Input: part model. Units: mm. Frame: model coordinates. A direction names the side the tool comes from. Give positions to 0.01 mm unless a question says otherwise; leave off trailing zeros. Loops run counter-clockwise (first coordinate to the right, second up) from the corner with the lowest first, then second, coordinate; pieces in that order, holes last. Notation, with made-up numbers: (85, 5) - (122, 5) arc R17 cw to (122, 19) - close; hole circle Ø4 at (59.5, 81.25). An arc over 180 degrees is marked (long way). One line per item, written item: value.
from build123d import *

# Parameters (mm, degrees)
F0_R     = 3.048
F0_R_2   = 2.54
F1_DEPTH = 3.937
F2_R     = 3.0417071759
F3_DEPTH = 0.635
F4_R     = 3.048
F5_DEPTH = 0.635
F6_SIZE2 = 0.50799
F6_SIZE  = 0.50799
F7_SIZE2 = 0.50799
F7_SIZE  = 0.50799


# Not quite as in the source:
# - a fillet or chamfer is up to 0.001 mm smaller than in the source, because OpenCascade refuses the exact size


with BuildPart() as f1:
    # F0 (on Top) → F1 (new body, symmetric)
    with BuildSketch(Plane.XY):
        with BuildLine():
            ThreePointArc((-40.9946195992, 14.3710068385), (-42.0464330806, 16.9103092103), (-44.5857354524, 17.9621226917))
            ThreePointArc((-44.5857354524, 17.9621226917), (-48.1768513056, 14.3710068385), (-44.5857354524, 10.7798909853))
            ThreePointArc((-44.5857354524, 10.7798909853), (-42.0464330806, 11.8317044667), (-40.9946195992, 14.3710068385))
        make_face()
        with Locations((-44.5857354524, 14.3710068385)):
            Circle(F0_R, mode=Mode.SUBTRACT)
        with BuildLine():
            ThreePointArc((-49.1226195992, 14.3710068385), (-50.1744330806, 16.9103092103), (-52.7137354524, 17.9621226917))
            ThreePointArc((-52.7137354524, 17.9621226917), (-56.3048513056, 14.3710068385), (-52.7137354524, 10.7798909853))
            ThreePointArc((-52.7137354524, 10.7798909853), (-50.1744330806, 11.8317044667), (-49.1226195992, 14.3710068385))
        make_face()
        with Locations((-52.7137354524, 14.3710068385)):
            Circle(F0_R, mode=Mode.SUBTRACT)
        with BuildLine():
            ThreePointArc((-32.8666195992, 14.3710068385), (-33.9184330806, 16.9103092103), (-36.4577354524, 17.9621226917))
            ThreePointArc((-36.4577354524, 17.9621226917), (-40.0488513056, 14.3710068385), (-36.4577354524, 10.7798909853))
            ThreePointArc((-36.4577354524, 10.7798909853), (-33.9184330806, 11.8317044667), (-32.8666195992, 14.3710068385))
        make_face()
        with Locations((-36.4577354524, 14.3710068385)):
            Circle(F0_R, mode=Mode.SUBTRACT)
        with BuildLine():
            ThreePointArc((-24.7386195992, 14.3710068385), (-25.7904330806, 16.9103092103), (-28.3297354524, 17.9621226917))
            ThreePointArc((-28.3297354524, 17.9621226917), (-31.9208513056, 14.3710068385), (-28.3297354524, 10.7798909853))
            ThreePointArc((-28.3297354524, 10.7798909853), (-25.7904330806, 11.8317044667), (-24.7386195992, 14.3710068385))
        make_face()
        with Locations((-28.3297354524, 14.3710068385)):
            Circle(F0_R, mode=Mode.SUBTRACT)
        with BuildLine():
            ThreePointArc((-60.8417354524, 10.7798909853), (-58.3024330806, 11.8317044667), (-57.2506195992, 14.3710068385))
            ThreePointArc((-57.2506195992, 14.3710068385), (-58.3024330806, 16.9103092103), (-60.8417354524, 17.9621226917))
            ThreePointArc((-60.8417354524, 17.9621226917), (-64.4328513056, 14.3710068385), (-60.8417354524, 10.7798909853))
        make_face()
        with Locations((-60.8417354524, 14.3710068385)):
            Circle(F0_R, mode=Mode.SUBTRACT)
        with Locations((-44.5857354524, 14.3710068385)):
            Circle(F0_R)
        with Locations((-44.5857354524, 14.3710068385)):
            Circle(F0_R_2, mode=Mode.SUBTRACT)
        with Locations((-36.4577354524, 14.3710068385)):
            Circle(F0_R)
        with Locations((-36.4577354524, 14.3710068385)):
            Circle(F0_R_2, mode=Mode.SUBTRACT)
        with Locations((-52.7137354524, 14.3710068385)):
            Circle(F0_R)
        with Locations((-52.7137354524, 14.3710068385)):
            Circle(F0_R_2, mode=Mode.SUBTRACT)
        with Locations((-28.3297354524, 14.3710068385)):
            Circle(F0_R)
        with Locations((-28.3297354524, 14.3710068385)):
            Circle(F0_R_2, mode=Mode.SUBTRACT)
        with Locations((-60.8417354524, 14.3710068385)):
            Circle(F0_R)
        with Locations((-60.8417354524, 14.3710068385)):
            Circle(F0_R_2, mode=Mode.SUBTRACT)
        with BuildLine():
            ThreePointArc((-60.8417354524, 17.9621226917), (-58.3024330806, 16.9103092103), (-57.2506195992, 14.3710068385))
            ThreePointArc((-57.2506195992, 14.3710068385), (-58.3024330806, 11.8317044667), (-60.8417354524, 10.7798909853))
            Line((-60.8417354524, 10.7798909853), (-52.7137354524, 10.7798909853))
            ThreePointArc((-52.7137354524, 10.7798909853), (-56.3048513056, 14.3710068385), (-52.7137354524, 17.9621226917))
            Line((-52.7137354524, 17.9621226917), (-60.8417354524, 17.9621226917))
        make_face()
        with BuildLine():
            Line((-44.5857354524, 17.9621226917), (-52.7137354524, 17.9621226917))
            ThreePointArc((-52.7137354524, 17.9621226917), (-50.1744330806, 16.9103092103), (-49.1226195992, 14.3710068385))
            ThreePointArc((-49.1226195992, 14.3710068385), (-50.1744330806, 11.8317044667), (-52.7137354524, 10.7798909853))
            Line((-52.7137354524, 10.7798909853), (-44.5857354524, 10.7798909853))
            ThreePointArc((-44.5857354524, 10.7798909853), (-48.1768513056, 14.3710068385), (-44.5857354524, 17.9621226917))
        make_face()
        with BuildLine():
            Line((-28.3297354524, 17.9621226917), (-36.4577354524, 17.9621226917))
            ThreePointArc((-36.4577354524, 17.9621226917), (-33.9184330806, 16.9103092103), (-32.8666195992, 14.3710068385))
            ThreePointArc((-32.8666195992, 14.3710068385), (-33.9184330806, 11.8317044667), (-36.4577354524, 10.7798909853))
            Line((-36.4577354524, 10.7798909853), (-28.3297354524, 10.7798909853))
            ThreePointArc((-28.3297354524, 10.7798909853), (-31.9208513056, 14.3710068385), (-28.3297354524, 17.9621226917))
        make_face()
        with BuildLine():
            Line((-36.4577354524, 17.9621226917), (-44.5857354524, 17.9621226917))
            ThreePointArc((-44.5857354524, 17.9621226917), (-42.0464330806, 16.9103092103), (-40.9946195992, 14.3710068385))
            ThreePointArc((-40.9946195992, 14.3710068385), (-42.0464330806, 11.8317044667), (-44.5857354524, 10.7798909853))
            Line((-44.5857354524, 10.7798909853), (-36.4577354524, 10.7798909853))
            ThreePointArc((-36.4577354524, 10.7798909853), (-40.0488513056, 14.3710068385), (-36.4577354524, 17.9621226917))
        make_face()
    extrude(amount=F1_DEPTH, both=True)

    # F2 (on face) → F3 (cut)
    with BuildSketch(Plane.XY.offset(3.937)):
        with Locations((-28.3297354524, 14.3710068385)):
            Circle(F2_R)
        with Locations((-36.4577354524, 14.3710068385)):
            Circle(F2_R)
        with Locations((-44.5857354524, 14.3710068385)):
            Circle(F2_R)
        with Locations((-52.7137354524, 14.3710068385)):
            Circle(F2_R)
        with Locations((-60.8417354524, 14.3710068385)):
            Circle(F2_R)
    extrude(amount=-F3_DEPTH, mode=Mode.SUBTRACT)

    # F4 (on face) → F5 (cut)
    with BuildSketch(Plane(origin=(0, 0, -3.937), x_dir=(1, 0, 0), z_dir=(0, 0, -1))):
        with Locations((-60.8417354524, -14.3710068385)):
            Circle(F4_R)
        with Locations((-52.7137354524, -14.3710068385)):
            Circle(F4_R)
        with Locations((-44.5857354524, -14.3710068385)):
            Circle(F4_R)
        with Locations((-36.4577354524, -14.3710068385)):
            Circle(F4_R)
        with Locations((-28.3297354524, -14.3710068385)):
            Circle(F4_R)
    extrude(amount=-F5_DEPTH, mode=Mode.SUBTRACT)

    # F6 (size 0.508 and 0.508 in the source; OpenCascade refuses exactly that, so slightly less here)
    f6_edges = [f1.edges().sort_by_distance(p)[0] for p in [
        (-38.997735, 14.371007, -3.302),
    ]]
    chamfer(f6_edges, length=F6_SIZE, length2=F6_SIZE2)

    # F7 (size 0.508 and 0.508 in the source; OpenCascade refuses exactly that, so slightly less here)
    f7_edges = [f1.edges().sort_by_distance(p)[0] for p in [
        (-47.125735, 14.371007, -3.302),
        (-55.253735, 14.371007, -3.302),
        (-63.381735, 14.371007, -3.302),
        (-30.869735, 14.371007, -3.302),
    ]]
    chamfer(f7_edges, length=F7_SIZE, length2=F7_SIZE2)


solid = f1.part
Item 1: Draft query along Y for faces 4 (the face through (-44, 17.962, 0)), 5 (the face through (-33.642, 15.538, -3.624)), 6 (the face through (-45, 10.78, 0)). Return one class per face: pulls with the +Y half, pulls with the -Y half, needs draft (parallel to the pull), parting line crosses it, or undercut.
Verdict:
face 4: pulls with the +Y half
face 5: undercut
face 6: pulls with the -Y half
Item 2: Section A-A, the plane z = 1.75. Output: boundary loops of the cut face in (x, y).
Verdict:
outline: (-60.84, 10.78) - (-28.33, 10.78) arc R3.59 ccw to (-28.33, 17.96) - (-60.84, 17.96) arc R3.59 ccw to start; hole circle Ø5.08 at (-60.84, 14.37); hole circle Ø5.08 at (-52.71, 14.37); hole circle Ø5.08 at (-44.59, 14.37); hole circle Ø5.08 at (-36.46, 14.37); hole circle Ø5.08 at (-28.33, 14.37)
Item 3: Section B-B, the plane y = 15. Count the separate pieces of the cut face and the enclosed holes in it, and give its area (3 significant figures).
Verdict:
separate pieces: 6
enclosed holes: 0
area: 110 mm^2
Item 4: Access query for faces 1 (the face through (-58.419, 15.134, 0.211)), 2 (the face through (-55.128, 12.52, 3.624)), 3 (the face through (-55.76, 14.24, -3.62)). Directions: +Z, -Z, +X, -X, +Y, -Y. A direction counts if a zero-diameter tool reaches every point of the face in a straight line with its end or side. Return the directions, or none.
Verdict:
face 1: +Z, -Z
face 2: +Z
face 3: -Z
Item 5: Material intervals for L1, parallel to X at y = 12.25, z = -1.25; L2, parallel to X at y = 14, z = -3.5; L3, parallel to Y at x = -30.5, z = -0.75, sorted ascending.
Verdict:
L1: x = -63.74 to -62.24, -59.44 to -54.11, -51.32 to -45.98, -43.19 to -37.86, -35.06 to -29.73, -26.93 to -25.43
L2: x = -64.41 to -63.87, -57.82 to -55.74, -49.69 to -47.61, -41.56 to -39.48, -33.43 to -31.36, -25.3 to -24.76
L3: y = 10.78 to 13.05, 15.69 to 17.96
Item 6: Pin query (flat end, axial travel): P1, Ø2, axis at y = 15.5, z = 0, coming from the -X side; P2, Ø2, axis at y = 16.5, z = -2.5, coming from the +X side; P3, Ø4, axis at x = -44.59, y = 14.37, coming from the -Z side. Return the tip coordinate at first contact, or that it passes through.
Verdict:
P1: stops at x = -64.43
P2: stops at x = -24.92
P3: passes through
